Verification items for the finished model (mm, model axes). Coordinates: 2 decimals unless noted, no trailing zeros. Order: outer loops, then holes, each group sorted by start corner. A loop starts at its lowest first (then second) coordinate and runs counter-clockwise, first axis right, second up. Notation, with made-up numbers: M 77.5,83 L 93.5,83 A3 ccw 93.5,88 Z; hole C 17,19 d11. An arc over 180 degrees is marked long. Return JSON: item names as keys, results as strings. Group by question number.
Q1. Section check C-C, the plane x = 2.5. Enter the section's corners in (y, z).
Q2. Section check B-B, the plane y = -5.75. Enter the section's corners in (x, z), then the cut area to 3 significant figures.
Q3. Mould release check, pull along X, two halves, no side actions. Record for faces 1 (the face through (58, -5, 0)), 2 (the face through (24, -10, 0)), 3 (the face through (46.86, -5.07, 1.3)): pulls with the +X half, pulls with the -X half, needs draft (parallel to the pull), parting line crosses it, or undercut.
Q4. Section check A-A, the plane z = 0. Enter the section's corners in (x, y).
Q5. Section check D-D, the plane x = 26.5. Enter the section's corners in (y, z).
Q6. Thickness scan on probe 1 along Z at (x, y) = (0, -7.5); probe 2 along X at (y, z) = (-8.5, -0.75); probe 3 along X at (y, z) = (-5.5, 0.5). Record the ranges inside material, lowest first.
Q7. Go/stop test with flat-tipped pins: pin 1 Ø4 at (x, y) = (-1.5, -2.5) entering from +Z; pin 2 Ø1.5 at (x, y) = (28.5, -4.5) entering from -Z; pin 3 Ø4 at (y, z) = (-7, 4) entering from +X; pin 4 Ø3 at (x, y) = (34.5, -8) entering from +Z. Record where each tip stops, or that it passes through.
from build123d import *

# Parameters (mm, degrees)
F1_DEPTH = 10
F2_D     = 10.8
F3_D     = 6.8


with BuildPart() as f1:
    # F0 (on Front) → F1 (new body)
    with BuildSketch(Plane.XZ):
        with BuildLine():
            Line((50.32, 7.9935974379), (0.4, 9.9919967974))
            ThreePointArc((0.4, 9.9919967974), (-10, 0), (0.4, -9.9919967974))
            Line((0.4, -9.9919967974), (50.32, -7.9935974379))
            ThreePointArc((50.32, -7.9935974379), (58, 0), (50.32, 7.9935974379))
        make_face()
    extrude(amount=F1_DEPTH)

    # F2 (through all)
    with Locations(Plane(origin=(0, 0, 0), x_dir=(1, 0, 0), z_dir=(0, 1, 0))):
        with Locations((0, 0)):
            Hole(F2_D / 2)

    # F3 (through all)
    with Locations(Plane(origin=(0, 0, 0), x_dir=(1, 0, 0), z_dir=(0, 1, 0))):
        with Locations((50, 0)):
            Hole(F3_D / 2)


solid = f1.part
Numbers:
{
 "1": {"outline": "M -10,-9.91 L 0,-9.91 L 0,-4.79 L -10,-4.79 Z; M -10,4.79 L 0,4.79 L 0,9.91 L -10,9.91 Z"},
 "2": {"outline": "M 0.4,-9.99 L 50.32,-7.99 A8 ccw 50.32,7.99 L 0.4,9.99 A10 ccw long Z; hole C 0,0 d10.8; hole C 50,0 d6.8", "area": "1,030 mm2"},
 "3": {"face 1": "pulls with the +X half", "face 2": "needs draft", "face 3": "undercut"},
 "4": {"outline": "M -10,-10 L -5.4,-10 L -5.4,0 L -10,0 Z; M 5.4,-10 L 46.6,-10 L 46.6,0 L 5.4,0 Z; M 53.4,-10 L 58,-10 L 58,0 L 53.4,0 Z"},
 "5": {"outline": "M -10,-8.95 L 0,-8.95 L 0,8.95 L -10,8.95 Z"},
 "6": {"probe 1": "z = -10 to -5.4, 5.4 to 10", "probe 2": "x = -9.97 to -5.35, 5.35 to 46.68, 53.32 to 57.96", "probe 3": "x = -9.99 to -5.38, 5.38 to 46.64, 53.36 to 57.98"},
 "7": {"pin 1": "stops at z = 10", "pin 2": "stops at z = -8.9", "pin 3": "stops at x = 57.75", "pin 4": "stops at z = 8.69"}
}
